```python
from build123d import *

# Parameters (mm, degrees)
F1_DEPTH = 21.336
F2_R     = 6.8636528609
F3_DEPTH = 48.006
F3_TAPER = 3


with BuildPart() as f1:
    # F0 (on Top) → F1 (new body)
    with BuildSketch(Plane.XY):
        Polygon((96.2734487839, 82.116805017), (-40.8865512161, 82.116805017), (-40.8865512161, 27.7571524011), (0, 0), (37.7825030637, 0), (96.2734487839, 34.8460475412), align=None)
        Polygon((89.9234488606, 75.7668050937), (89.9234488606, 38.4544916451), (36.0343505215, 6.3499999233), (1.9518097804, 6.3499999233), (-34.5365512928, 31.1212992638), (-34.5365512928, 75.7668050937), align=None, mode=Mode.SUBTRACT)
    extrude(amount=F1_DEPTH)

    # F2 (on Top) → F3 (join)
    with BuildSketch(Plane.XY):
        Circle(F2_R)
        with Locations((38.1801947951, 0)):
            Circle(F2_R)
        with Locations((96.5343341231, 82.1052864194)):
            Circle(F2_R)
        with Locations((-40.7790951431, 27.5509990752)):
            Circle(F2_R)
    extrude(amount=F3_DEPTH, taper=F3_TAPER)


solid = f1.part
```
Geometry check sheet. Reference: the model listing, model coordinates, mm. A direction names the side the tool comes from. Coordinates: 2 decimals unless noted, no trailing zeros. Loops run counter-clockwise (first coordinate to the right, second up) from the corner with the lowest first, then second, coordinate; pieces in that order, holes last. Notation, with made-up numbers: (-19, 48) - (34, 48) arc R13 ccw to (34, 54) - close; hole circle Ø9 at (42.25, 73). An arc over 180 degrees is marked (long way). One line per item, written item: value. Start each with the question number.
(1) Cross-section at B-B on y = 47.5. Enter the section's corners in (x, z).
(2) Mould release check, pull along Y, two halves, no side actions. Record for faces 3 (the conical face through (-45.214, 24.151, 24.339)), 4 (the flat face through (28, 77, 0)), 5 (the flat face through (-34.537, 53, 11)): released by +Y, released by -Y, zero draft, split by the parting line, or undercut.
(3) Cross-section at A-A on x = 23. Enter the section's corners in (y, z), plus the area to 3 significant figures.
(4) Depth check by flat-ended pin: P1, Ø17, axis at y = 57.5, z = 11.5, coming from the -X side; P2, Ø6.5, axis at x = 12, z = 8, coming from the -Y side; P3, Ø23.5, axis at x = 10.5, z = 13, coming from the +Y side; P4, Ø10, axis at y = 68, z = 35.5, coming from the +X side. Enter the tip coordinate at first touch or a pass-through.
(5) Cross-section at C-C on z = 7. Enter the section's corners in (x, y), plus the area to 3 significant figures.
(6) Tool access check on faces 1 (the flat face through (63.36, 22.63, 10.52)), 2 (the flat face through (0, 0, 48.006)). Record the directions out of +Z, -Z, +X, -X, +Y, -Y that give a thin tool (end or side, any length) a straight path to the whole face; none if there is none.
(7) Material ranges on line 1 (Y direction, x = 26.5, z = 12.5); line 2 (X direction, y = 73, z = 14); line 3 (Y direction, x = 33.5, z = 3.5), recorded low to high. Write a range as [from, to].
Results below:
1. outline: (-40.89, 0) - (-34.54, 0) - (-34.54, 21.34) - (-40.89, 21.34) - close; (89.92, 0) - (96.27, 0) - (96.27, 21.34) - (89.92, 21.34) - close
2. face 3: split by the parting line
2. face 4: zero draft
2. face 5: undercut
3. outline: (0, 0) - (6.35, 0) - (6.35, 21.34) - (0, 21.34) - close; (75.77, 0) - (82.12, 0) - (82.12, 21.34) - (75.77, 21.34) - close
3. area: 271 mm2
4. P1: stops at x = -40.89
4. P2: stops at y = 0
4. P3: stops at y = 82.12
4. P4: passes through
5. outline: (-40.89, 34.05) arc R6.5 ccw (long way) to (-35.34, 23.99) - (-5.38, 3.65) arc R6.5 ccw (long way) to (6.5, 0) - (31.68, 0) arc R6.5 ccw (long way) to (43.65, 3.5) - (96.27, 34.85) - (96.27, 75.61) arc R6.5 ccw (long way) to (90.04, 82.12) - (-40.89, 82.12) - close; hole (-34.54, 31.12) - (1.95, 6.35) - (36.03, 6.35) - (89.92, 38.45) - (89.92, 75.77) - (-34.54, 75.77) - close
5. area: 2,700 mm2
6. face 1: +Z, -Z
6. face 2: +Z, +X, -X, +Y, -Y
7. line 1: y = [0, 6.35], [75.77, 82.12]
7. line 2: x = [-40.89, -34.54], [89.92, 96.27]
7. line 3: y = [-4.77, 6.35], [75.77, 82.12]
